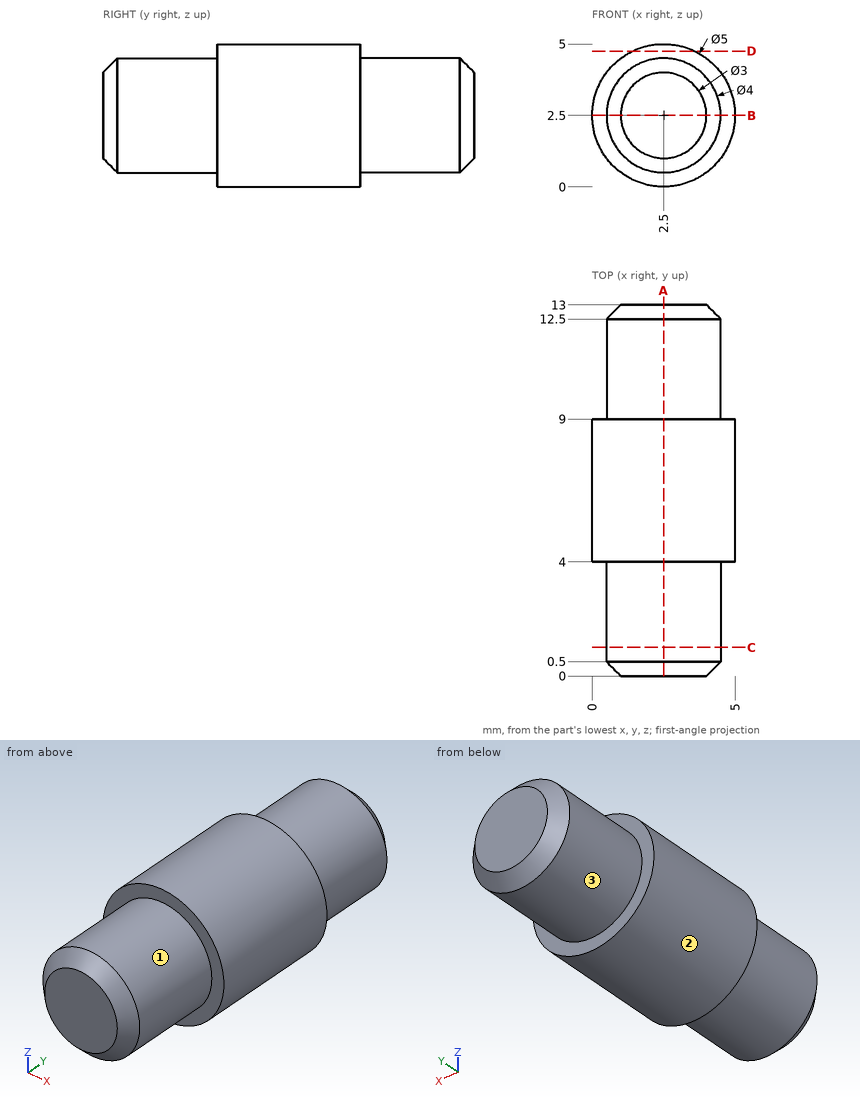
Input: dimensioned drawing with shaded views. Units: mm. Origin: part minimum x, y, z. A direction names the side the tool comes from. Coordinates: 2 decimals unless noted, no trailing zeros. Loops run counter-clockwise (first coordinate to the right, second up) from the corner with the lowest first, then second, coordinate; pieces in that order, holes last. Notation, with made-up numbers: M -3.5,71 L 54.5,71 A19 ccw 54.5,80 Z; hole C -3,-24 d11. An arc over 180 degrees is marked long. One line per item, written item: value. Start each with the question number.
1) Reachability of the marked faces 1, 2 and 3 from +Z, -Z, +X, -X, +Y, -Y: full face, straight path, thin tool, end or side. Return the list, or none.
2) Pin query (flat end, axial travel): P1, Ø1.5, axis at x = 3.5, y = 6.5, coming from the -Z side; P2, Ø3, axis at x = 3, y = 3.5, coming from the +Z side; P3, Ø1.5, axis at x = 2.5, y = 11.5, coming from the +Z side. Return the tip coordinate at first contact, or that it passes through.
3) Cut plane B-B (z = 2.5). Return loops of the section in (x, y), then the cut area to 3 significant figures.
4) Cut plane D-D (z = 4.75). Return loops of the section in (x, y), then the cut area to 3 significant figures.
5) Cut plane C-C (y = 1). Return loops of the section in (x, z), then the cut area to 3 significant figures.
6) Cut plane A-A (x = 2.5). Return loops of the section in (y, z), then the cut area to 3 significant figures.
7) Material intervals for L1, parallel to Y at x = 4.15, z = 1.2; L2, parallel to X at y = 5.75, z = 2.8; L3, parallel to X at y = 6.75, z = 1.35, sorted ascending. Write a range as from..to.
Evaluation:
1. face 1: -Y
1. face 2: +Y, -Y
1. face 3: +Y
2. P1: z = 0.01
2. P2: z = 5
2. P3: z = 4.5
3. outline: M 0,4 L 0.5,4 L 0.5,0.5 L 1,0 L 4,0 L 4.5,0.5 L 4.5,4 L 5,4 L 5,9 L 4.5,9 L 4.5,12.5 L 4,13 L 1,13 L 0.5,12.5 L 0.5,9 L 0,9 Z
3. area: 56.5 mm^2
4. outline: M 1.41,4 L 3.59,4 L 3.59,9 L 1.41,9 Z
4. area: 10.9 mm^2
5. outline: C 2.5,2.5 d4
5. area: 12.6 mm^2
6. outline: M 0,1 L 0.5,0.5 L 4,0.5 L 4,0 L 9,0 L 9,0.5 L 12.5,0.5 L 13,1 L 13,4 L 12.5,4.5 L 9,4.5 L 9,5 L 4,5 L 4,4.5 L 0.5,4.5 L 0,4 Z
6. area: 56.5 mm^2
7. L1: 4..9
7. L2: 0.02..4.98
7. L3: 0.28..4.72
